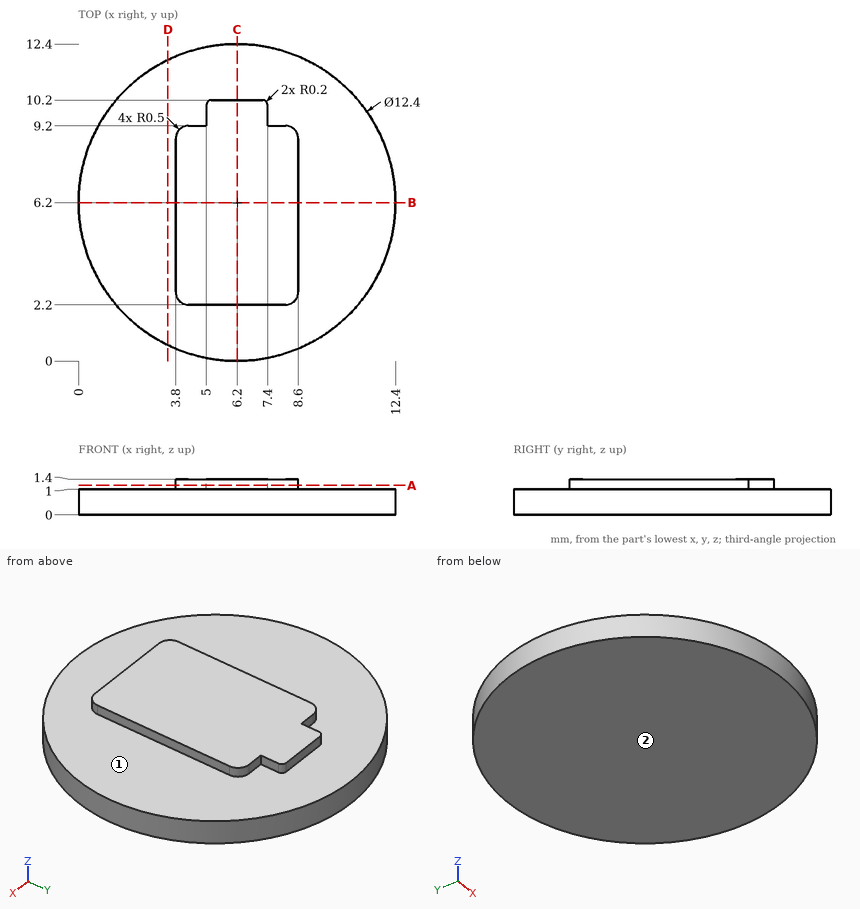
Verification items for this drawing (mm, ordinates from the low corner). A direction names the side the tool comes from. Round coordinates to 2 decimals unless told otherwise and drop trailing zeros. Write each loop counter-clockwise with the first axis right and the second up, starting at its lowest first coordinate (ties: lowest second). Pieces come first, ordered by that corner, then holes. Notation, with made-up numbers: (-31.5, 26.25) - (-14.5, 26.25) arc R20 ccw to (-14.5, 54.25) - close; hole circle Ø4 at (-2.5, 68.5). An arc over 180 degrees is marked (long way). Answer as a JSON object with one key per item and string values. Group by question number.
Q1. Tool access check on the marked faces 1 and 2. Record the directions out of +Z, -Z, +X, -X, +Y, -Y that give a thin tool (end or side, any length) a straight path to the whole face; none if there is none.
Q2. Thickness scan on line 1 (Y direction, x = 6, z = 1.1); line 2 (Z direction, x = 11.25, y = 5); line 3 (X direction, y = 8.5, z = 1.2). Record the ranges inside material, lowest first.
Q3. Section check D-D, the plane x = 3.5. Enter the section's corners in (y, z), plus the area to 3 significant figures.
Q4. Section check A-A, the plane z = 1.15. Enter the section's corners in (x, y).
Q5. Section check B-B, the plane y = 6.2. Enter the section's corners in (x, z), plus the area to 3 significant figures.
Q6. Section check C-C, the plane x = 6.2. Enter the section's corners in (y, z).
Found:
{
 "1": {"face 1": "+Z", "face 2": "-Z, +X, -X, +Y, -Y"},
 "2": {"line 1": "y = 2.2 to 10.2", "line 2": "z = 0 to 1", "line 3": "x = 3.8 to 8.6"},
 "3": {"outline": "(0.62, 0) - (11.78, 0) - (11.78, 1) - (0.62, 1) - close", "area": "11.2 mm^2"},
 "4": {"outline": "(3.8, 2.7) arc R0.5 ccw to (4.3, 2.2) - (8.1, 2.2) arc R0.5 ccw to (8.6, 2.7) - (8.6, 8.7) arc R0.5 ccw to (8.1, 9.2) - (7.4, 9.2) - (7.4, 10) arc R0.2 ccw to (7.2, 10.2) - (5.2, 10.2) arc R0.2 ccw to (5, 10) - (5, 9.2) - (4.3, 9.2) arc R0.5 ccw to (3.8, 8.7) - close"},
 "5": {"outline": "(0, 0) - (12.4, 0) - (12.4, 1) - (8.6, 1) - (8.6, 1.4) - (3.8, 1.4) - (3.8, 1) - (0, 1) - close", "area": "14.3 mm^2"},
 "6": {"outline": "(0, 0) - (12.4, 0) - (12.4, 1) - (10.2, 1) - (10.2, 1.4) - (2.2, 1.4) - (2.2, 1) - (0, 1) - close"}
}
